Source: three-view drawing plus pictorial views. Frame: mm from the lowest corner of the part. Coordinates: 2 decimals unless noted, no trailing zeros. Write each loop counter-clockwise with the first axis right and the second up, starting at its lowest first coordinate (ties: lowest second). Pieces come first, ordered by that corner, then holes. Notation, with made-up numbers: (24.5, 74.5) -> (56.5, 74.5) arc R21 cw to (56.5, 108.5) -> close; hole circle Ø4 at (54, -13). An arc over 180 degrees is marked (long way). One line per item, written item: value.
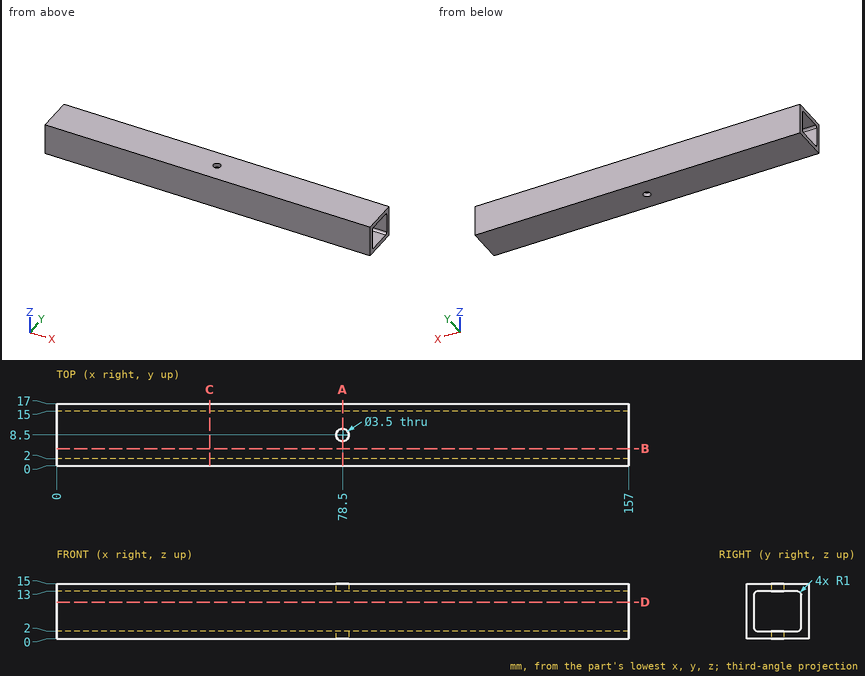
(1) Section C-C (x = 42). Return the cut outline in (y, z), then the cut area to 3 significant figures.
Responses:
outline: (0, 0) -> (17, 0) -> (17, 15) -> (0, 15) -> close; hole (2, 3) arc R1 ccw to (3, 2) -> (14, 2) arc R1 ccw to (15, 3) -> (15, 12) arc R1 ccw to (14, 13) -> (3, 13) arc R1 ccw to (2, 12) -> close
area: 113 mm2
(2) Section D-D (z = 10). Return the cut outline in (x, y).
Responses:
outline: (0, 0) -> (157, 0) -> (157, 2) -> (0, 2) -> close; (0, 15) -> (157, 15) -> (157, 17) -> (0, 17) -> close
(3) First-contact query: pin 1 (6 mm diameter, centred on x = 137.5, y = 7.5, fed in from -Z). Flat tip, straight axial feed; report the tip coordinate or a pass-through.
Responses:
pin 1: stops at z = 0
(4) Line query: line 1 (Z direction, x = 31.5, y = 12.75); line 2 (Y direction, x = 78.5, z = 0.7); line 3 (X direction, y = 8.5, z = 1.55). Output: solid intervals per line, ascending. Write a range as [from, to].
Responses:
line 1: z = [0, 2], [13, 15]
line 2: y = [0, 6.75], [10.25, 17]
line 3: x = [0, 76.75], [80.25, 157]
(5) Section A-A (x = 78.5). Return the cut outline in (y, z), then the cut area to 3 significant figures.
Responses:
outline: (0, 0) -> (6.75, 0) -> (6.75, 2) -> (3, 2) arc R1 cw to (2, 3) -> (2, 12) arc R1 cw to (3, 13) -> (6.75, 13) -> (6.75, 15) -> (0, 15) -> close; (10.25, 0) -> (17, 0) -> (17, 15) -> (10.25, 15) -> (10.25, 13) -> (14, 13) arc R1 cw to (15, 12) -> (15, 3) arc R1 cw to (14, 2) -> (10.25, 2) -> close
area: 98.9 mm2
(6) Section B-B (y = 4.75). Return the cut outline in (x, z), then the cut area to 3 significant figures.
Responses:
outline: (0, 0) -> (157, 0) -> (157, 2) -> (0, 2) -> close; (0, 13) -> (157, 13) -> (157, 15) -> (0, 15) -> close
area: 628 mm2
